Work out the finished part from the listing and answer in its coordinate system (mm). Face numbers are marked on the shaded views. A direction names the side the tool comes from. Coordinates: 2 decimals unless noted, no trailing zeros. Write each loop counter-clockwise with the first axis right and the second up, starting at its lowest first coordinate (ties: lowest second). Pieces come first, ordered by that corner, then holes. Notation, with made-up numbers: (33.25, 15) - (63.25, 15) arc R30 ccw to (63.25, 54) - close; hole circle Ø10 at (84.25, 74). An arc over 180 degrees is marked (long way). One line per item, written item: value.
```python
from build123d import *

# Parameters (mm, degrees)
BOSS_EXTRUDE1_DEPTH      = 12.7
BOSS_EXTRUDE2_DEPTH      = 3.175
BOSS_EXTRUDE2_DEPTH_BACK = 15.875
SKETCH3_R                = 1.524
SKETCH2_R                = 3.175
CUT_EXTRUDE1_DEPTH       = 55.869487053


with BuildPart() as part:
    # Sketch1 → Boss-Extrude1 (new body)
    with BuildSketch(Plane.XY):
        with BuildLine():
            Line((5.715, -5.715), (43.815, -5.715))
            Line((43.815, -5.715), (43.815, 5.715))
            Line((43.815, 5.715), (5.715, 5.715))
            Line((5.715, 5.715), (-5.715, 5.715))
            ThreePointArc((-5.715, 5.715), (-5.715, -5.715), (5.715, -5.715))
        make_face()
    extrude(amount=BOSS_EXTRUDE1_DEPTH)

    # Sketch3 → Boss-Extrude2 (add, two sides: drawn at the far end of the back side and taken through both)
    with BuildSketch(Plane.XY.offset(12.7).offset(-BOSS_EXTRUDE2_DEPTH_BACK)):
        Circle(SKETCH3_R)
    extrude(amount=BOSS_EXTRUDE2_DEPTH + BOSS_EXTRUDE2_DEPTH_BACK)

    # Sketch2 → Cut-Extrude1 (cut, through all)
    with BuildSketch(Plane(origin=(43.815, 0, 0), x_dir=(0, 0, -1), z_dir=(1, 0, 0))):
        with Locations((-6.35, 0)):
            Circle(SKETCH2_R)
    extrude(amount=-CUT_EXTRUDE1_DEPTH, mode=Mode.SUBTRACT)


solid = part.part
```
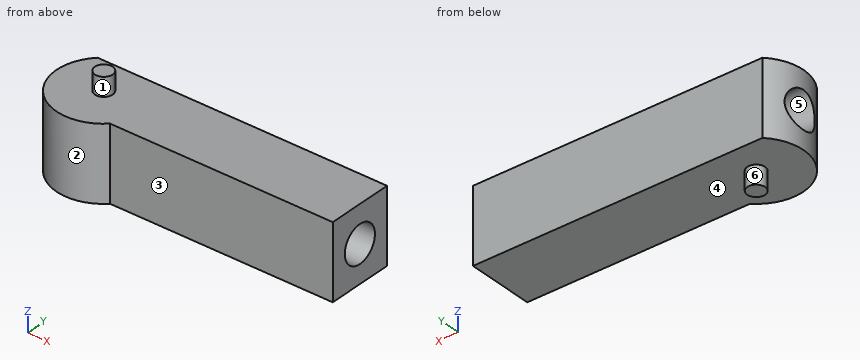
Item 1: Section D-D, the plane z = 6.35 is taken. Determine the outline of the cut face in (x, y) (3 decimals).
Evaluation:
outline: (-7.432, -3.175) arc R8.082 ccw to (5.715, -5.715) - (43.815, -5.715) - (43.815, -3.175) - close; (-7.432, 3.175) - (43.815, 3.175) - (43.815, 5.715) - (-5.715, 5.715) arc R8.082 ccw to start
Item 2: Section C-C, the plane z = 8.5 is taken. Determine the outline of the cut face in (x, y) (3 decimals), then the cut area to 3 significant figures.
Evaluation:
outline: (-7.737, -2.336) arc R8.082 ccw to (5.715, -5.715) - (43.815, -5.715) - (43.815, -2.336) - close; (-7.737, 2.336) - (43.815, 2.336) - (43.815, 5.715) - (-5.715, 5.715) arc R8.082 ccw to start
area: 361 mm2
Item 3: Section B-B, the plane y = 0 is taken. Determine the outline of the cut face in (x, z) (3 decimals).
Evaluation:
outline: (-8.082, 0) - (-1.524, 0) - (-1.524, -3.175) - (1.524, -3.175) - (1.524, 0) - (43.815, 0) - (43.815, 3.175) - (-8.082, 3.175) - close; (-8.082, 9.525) - (43.815, 9.525) - (43.815, 12.7) - (1.524, 12.7) - (1.524, 15.875) - (-1.524, 15.875) - (-1.524, 12.7) - (-8.082, 12.7) - close
Item 4: Section A-A, the plane x = 0 is taken. Determine the outline of the cut face in (y, z) (3 decimals).
Evaluation:
outline: (-8.082, 0) - (-1.524, 0) - (-1.524, -3.175) - (1.524, -3.175) - (1.524, 0) - (5.715, 0) - (5.715, 12.7) - (1.524, 12.7) - (1.524, 15.875) - (-1.524, 15.875) - (-1.524, 12.7) - (-8.082, 12.7) - close; hole circle Ø6.35 at (0, 6.35)
Item 5: Given pin 1 (5 mm diameter, centred on x = 24.5, z = 12.5, fed in from -Y) (3 decimals); pin 2 (5 mm diameter, centred on x = 36, y = -1.5, fed in from +Z); pin 3 (5 mm diameter, centred on y = 0, z = 6.35, fed in from -X); pin 4 (7 mm diameter, centred on x = 23.5, y = -2.5, fed in from -Z), each flat-ended and moving along its own axis, determine where each tip first touches the part or whether it passes through.
Evaluation:
pin 1: stops at y = -5.715
pin 2: stops at z = 12.7
pin 3: passes through
pin 4: stops at z = 0
Item 6: Determine the mould class of the marked faces 4, 5 and 6 for opening direction Y: +Y half, -Y half, draft (parallel to the pull), parting line (faces both ways), or undercut.
Evaluation:
face 4: draft
face 5: undercut
face 6: parting line
Item 7: Consider probe 1 along Z at (x, y) = (26, 0) (3 decimals); probe 2 along Y at (x, z) = (29, 6.35) (3 decimals); probe 3 along Z at (x, y) = (21, 5). Determine where each line is inside the solid, lowest interval first.
Evaluation:
probe 1: z = 0 to 3.175, 9.525 to 12.7
probe 2: y = -5.715 to -3.175, 3.175 to 5.715
probe 3: z = 0 to 12.7
Item 8: Which of the six approach directions +Z, -Z, +X, -X, +Y, -Y give full straight-line access (tool end or side, diameter ignored) to the marked faces 1, 2 and 3?
Evaluation:
face 1: +Z
face 2: +Z, -Z
face 3: +Z, -Z, +X, -Y
